Source: CAD feature listing. Evaluate the final solid. Frame: model axes, mm. Coordinates: 2 decimals unless noted, no trailing zeros. Order: outer loops, then holes, each group sorted by start corner. A loop starts at its lowest first (then second) coordinate and runs counter-clockwise, first axis right, second up. Notation, with made-up numbers: (85, 22) - (126, 22) arc R33 ccw to (126, 55) - close; hole circle Ø6 at (29, 46). An arc over 180 degrees is marked (long way). One line per question, with ' | ' between items. Start each with the question number.
(1) Contact query for flat-ended pins moving along their axis: P1, Ø1.5, axis at y = 3.5, z = 39.5, coming from the -X side; P2, Ø4, axis at y = 4.5, z = 42, coming from the -X side; P3, Ø4, axis at x = 195, z = 36.5, coming from the -Y side. Output: stop coordinate, or through.
(2) Section A-A (x = 269.5). Return the cut outline in (y, z), then the cut area to 3 significant figures.
(3) Line query: line 1 along Z through (x, y) = (171.5, 8.75); line 2 along X through (y, z) = (0.75, 41); line 3 along X through (y, z) = (9.75, 41.5) (3 decimals). Output: solid intervals per line, ascending.
(4) Section B-B (z = 37.5). Return the cut outline in (x, y) (3 decimals).
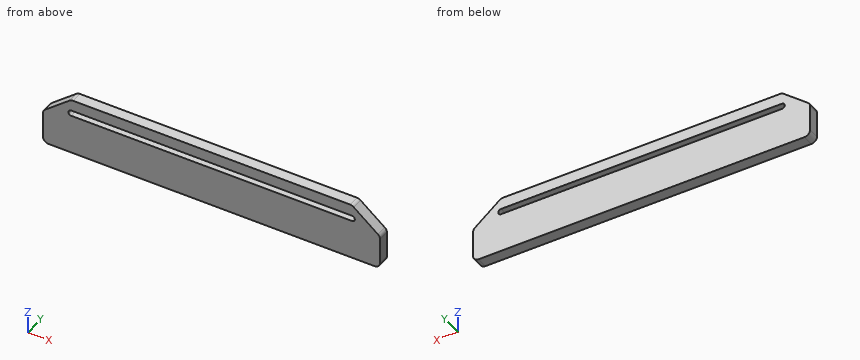
from build123d import *

# Parameters (mm, degrees)
BOSS_EXTRUDE1_DEPTH     = 10
CUT_EXTRUDE4_DEPTH      = 305.302481094
CUT_EXTRUDE4_DEPTH_BACK = 305.302481094


with BuildPart() as part:
    # Sketch1 → Boss-Extrude1 (new body)
    with BuildSketch(Plane(origin=(0, 0, 0), x_dir=(1, 0, 0), z_dir=(0, 1, 0))):
        with BuildLine():
            Line((0, -5), (0, -27.596875763))
            ThreePointArc((0, -27.596875763), (0.493483818, -29.762819415), (1.876524762, -31.50121981))
            Line((1.876524762, -31.50121981), (23.630430059, -48.904344047))
            ThreePointArc((23.630430059, -48.904344047), (25.09887059, -49.718141596), (26.753905297, -50))
            Line((26.753905297, -50), (273.246094703, -50))
            ThreePointArc((273.246094703, -50), (274.90112941, -49.718141596), (276.369569941, -48.904344047))
            Line((276.369569941, -48.904344047), (298.123475238, -31.50121981))
            ThreePointArc((298.123475238, -31.50121981), (299.506516182, -29.762819415), (300, -27.596875763))
            Line((300, -27.596875763), (300, -5))
            ThreePointArc((300, -5), (298.535533906, -1.464466094), (295, 0))
            Line((295, 0), (5, 0))
            ThreePointArc((5, 0), (1.464466094, -1.464466094), (0, -5))
        make_face()
    extrude(amount=BOSS_EXTRUDE1_DEPTH)

    # Sketch2 → Cut-Extrude4 (cut, two sides: drawn at the far end of the back side and taken through both)
    with BuildSketch(Plane(origin=(0, 0, 0), x_dir=(1, 0, 0), z_dir=(0, 1, 0)).offset(-CUT_EXTRUDE4_DEPTH_BACK)):
        with BuildLine():
            Line((25, -35), (275, -35))
            ThreePointArc((275, -35), (277.5, -37.5), (275, -40))
            Line((275, -40), (25, -40))
            ThreePointArc((25, -40), (22.5, -37.5), (25, -35))
        make_face()
    extrude(amount=CUT_EXTRUDE4_DEPTH + CUT_EXTRUDE4_DEPTH_BACK, mode=Mode.SUBTRACT)


solid = part.part
Response values:
1) P1: stops at x = 10.94 | P2: stops at x = 12.5 | P3: stops at y = 0
2) outline: (0, 0) - (10, 0) - (10, 35) - (0, 35) - close; (0, 40) - (10, 40) - (10, 50) - (0, 50) - close | area: 450 mm²
3) line 1: z = 0 to 35, 40 to 50 | line 2: x = 13.75 to 286.25 | line 3: x = 14.375 to 285.625
4) outline: (9.375, 0) - (22.5, 0) - (22.5, 10) - (9.375, 10) - close; (277.5, 0) - (290.625, 0) - (290.625, 10) - (277.5, 10) - close
